Autodesk Inventor part; units mm, degrees
ref_plane "YZ Plane" through (0, 0, 0) normal (1, 0, 0) x (0, 1, 0)
ref_plane "XZ Plane" through (0, 0, 0) normal (0, 1, 0) x (-1, 0, 0)
ref_plane "XY Plane" through (0, 0, 0) normal (0, 0, 1) x (1, 0, 0)
sketch "Skizze1" plane through (0, 0, 0) normal (0, 0, 1) x (1, 0, 0)
  line L0 (0, 0) -> (16.2131, 0)
  line L1 (0, 2) -> (17.5, 2)
  line L2 (17.5, 2) -> (17.5, 6)
  line L3 (17.5, 6) -> (13, 6)
  line L4 (13, 6) -> (13, 16)
  line L5 (13, 16) -> (9, 16)
  line L6 (9, 16) -> (9, 6)
  line L7 (9, 6) -> (0, 6)
  line L8 (0, 6) -> (0, 2)
  dimension "d0" = 4
  dimension "d1" = 9
  dimension "d2" = 2
  dimension "d3" = 4.5
  dimension "d4" = 10
  dimension "d5" = 0
  dimension "d6" = 4
  dimension "d8" = 1.2869
revolve "Umdrehung1" add sketch "Skizze1" angle 360 about axis through (0, 0, 0) along (1, 0, 0)
properties part number "Kupplung"
Can you work these out from the model? Positions are in its coordinate system, mm. A direction names the side the tool comes from. Give positions to 0.01 mm unless a question says otherwise; leave off trailing zeros. Write each loop counter-clockwise with the first axis right and the second up, starting at its lowest first coordinate (ties: lowest second). Pieces come first, ordered by that corner, then holes. Notation, with made-up numbers: (70, -2.5) -> (80, -2.5) arc R18 ccw to (80, 6.5) -> close; hole circle Ø2 at (21, 76.25). An arc over 180 degrees is marked (long way). Write item = value, one per line.
(1) I need wall thicknesses on probe 1 along Z at (x, y) = (4, 0); probe 2 along Z at (x, y) = (10.25, 0); probe 3 along X at (y, z) = (-12, 7.5). Which ranges of each line are inside material? Lowest first, please. Write a range as from..to.
Worked out:
probe_1 = -6..-2, 2..6
probe_2 = -16..-2, 2..16
probe_3 = 9..13
(2) Suppose I cut it at A-A on y = 0. Write out the boundary of the cut face in (x, z), then the cut area to 3 significant figures.
Worked out:
outline = (0, -6) -> (9, -6) -> (9, -16) -> (13, -16) -> (13, -6) -> (17.5, -6) -> (17.5, -2) -> (0, -2) -> close; (0, 2) -> (17.5, 2) -> (17.5, 6) -> (13, 6) -> (13, 16) -> (9, 16) -> (9, 6) -> (0, 6) -> close
area = 220 mm^2
(3) Suppose I cut it at C-C on x = 3.5. Write out the boundary of the cut face in (y, z).
Worked out:
outline = circle Ø12 at (0, 0); hole circle Ø4 at (0, 0)
(4) Suppose I cut it at D-D on z = 10. Write out the boundary of the cut face in (x, y), then the cut area to 3 significant figures.
Worked out:
outline = (9, -12.49) -> (13, -12.49) -> (13, 12.49) -> (9, 12.49) -> close
area = 99.9 mm^2
(5) I'm going to push flat-ended pins straight in: P1, Ø8, axis at x = 5.5, y = 3, coming from the -Z side; P2, Ø6, axis at x = 15, y = -3.5, coming from the +Z side; P3, Ø3, axis at x = 5, z = -4, coming from the -Y side. Where does each tip first touch, or does it pass through?
Worked out:
P1 = -15.96
P2 = 15.95
P3 = -5.45
(6) Thinking about a two-plate mould opening in Y: for faces 1 (the face through (13, 7, 0)), 2 (the face through (9, 0, -2)), 3 (the face through (10.97, -3.47, 15.62)), which applies, released by +Y, released by -Y, zero draft, split by the parting line, or undercut?
Worked out:
face_1 = zero draft
face_2 = undercut
face_3 = split by the parting line
(7) For faces 4 (the face through (15, -6, 0)), 5 (the face through (9, 7, 0)), 6 (the face through (0, 3, 0)), which set-ups out of +Z, -Z, +X, -X, +Y, -Y let a thin tool reach every point of the face, with its end or its side?
Worked out:
face_4 = +X
face_5 = -X
face_6 = +Z, -Z, -X, +Y, -Y
